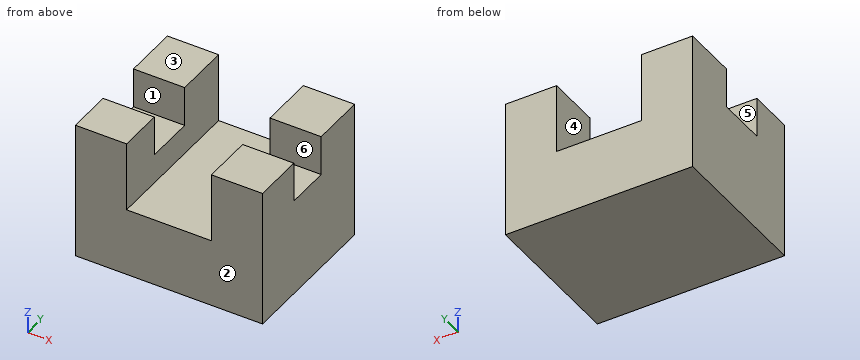
```python
from build123d import *

# Parameters (mm, degrees)
F1_DEPTH = 50.8
F2_W     = 17.3335857689
F2_H     = 15.0761622936
F3_DEPTH = 13.589
F4_W     = 17.3335857689
F4_H     = 16.7590361089
F5_DEPTH = 13.589


with BuildPart() as f1:
    # F0 (on Front) → F1 (new body)
    with BuildSketch(Plane.XZ):
        Polygon((0, 46.8351207674), (0, 0), (63.3651614189, 0), (63.3651614189, 46.8351207674), (46.03157565, 46.8351207674), (46.03157565, 23.1879781932), (17.3335857689, 23.1879781932), (17.3335857689, 46.8351207674), align=None)
    extrude(amount=F1_DEPTH)

    # F2 (on face) → F3 (cut)
    with BuildSketch(Plane.XY.offset(46.8351207674)):
        with Locations((54.6983685344, -25.9903585538)):
            Rectangle(F2_W, F2_H)
    extrude(amount=-F3_DEPTH, mode=Mode.SUBTRACT)

    # F4 (on face) → F5 (cut)
    with BuildSketch(Plane.XY.offset(46.8351207674)):
        with Locations((8.6667928845, -27.1185943857)):
            Rectangle(F4_W, F4_H)
    extrude(amount=-F5_DEPTH, mode=Mode.SUBTRACT)


solid = f1.part
```
The model under review builds one solid part; all positions refer to its coordinate system, in mm. Face numbers are marked on the shaded views. A direction names the side the tool comes from. Round coordinates to 2 decimals unless told otherwise and drop trailing zeros. Loops run counter-clockwise (first coordinate to the right, second up) from the corner with the lowest first, then second, coordinate; pieces in that order, holes last. Notation, with made-up numbers: M 41,44.25 L 79,44.25 A25 cw 79,71.25 Z; hole C 13.5,23 d4. An arc over 180 degrees is marked long. Write item = value, one per line.
Item 1: Take a section at C-C on x = 8. Write out the cut boundary in (y, z).
Return value:
outline = M -50.8,0 L 0,0 L 0,46.84 L -18.74,46.84 L -18.74,33.25 L -35.5,33.25 L -35.5,46.84 L -50.8,46.84 Z
Item 2: For line 1 (X direction, y = -21.5, z = 28); line 2 (Z direction, x = 44, y = -37); line 3 (Z direction, x = 13.5, y = -19), list the stretches that pass through material, from the lowest coordinate up. Write a range as [from, to].
Return value:
line_1 = [0, 17.33], [46.03, 63.37]
line_2 = [0, 23.19]
line_3 = [0, 33.25]
Item 3: Take a section at B-B on y = -28.5. Write out the cut boundary in (x, z).
Return value:
outline = M 0,0 L 63.37,0 L 63.37,33.25 L 46.03,33.25 L 46.03,23.19 L 17.33,23.19 L 17.33,33.25 L 0,33.25 Z
Item 4: The part is to be moulded in two halves that separate along Y. For the marked faces 1, 2 and 3, say which applies: released by +Y, released by -Y, zero draft, split by the parting line, or undercut.
Return value:
face_1 = undercut
face_2 = released by -Y
face_3 = zero draft
Item 5: Take a section at D-D on x = 28.5. Write out the cut boundary in (y, z).
Return value:
outline = M -50.8,0 L 0,0 L 0,23.19 L -50.8,23.19 Z
Item 6: Take a section at A-A on z = 29. Write out the cut boundary in (x, y).
Return value:
outline = M 0,-50.8 L 17.33,-50.8 L 17.33,0 L 0,0 Z; M 46.03,-50.8 L 63.37,-50.8 L 63.37,0 L 46.03,0 Z
Item 7: Insertion check: P1, Ø11, axis at x = 51.5, z = 43, coming from the +Y side; P2, Ø4.5, axis at x = 52.5, y = -25, coming from the +Z side. Each pin has a flat end and moves straight along its axis. Give the tip position at first contact, or say it passes through.
Return value:
P1 = 0
P2 = 33.25
Item 8: Machinability: for the marked faces 4, 5 and 6, which of the approach directions +Z, -Z, +X, -X, +Y, -Y give a long, thin tool a straight path to every point of the face, cutting with its end or side? Answer none if there is none.
Return value:
face_4 = +Z, +Y, -Y
face_5 = +Z, -X
face_6 = +Z, +X
